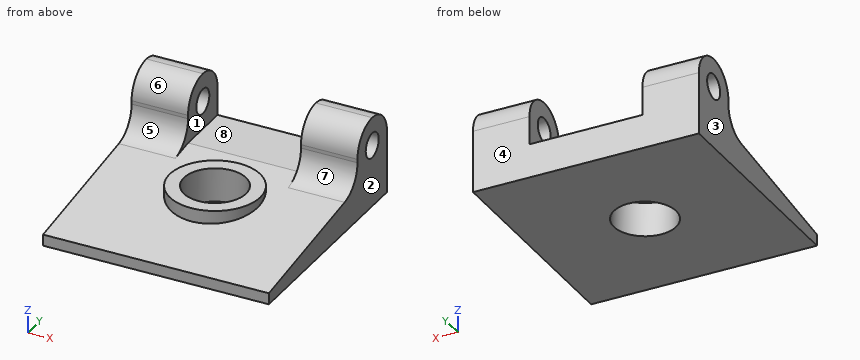
from build123d import *

# Parameters (mm, degrees)
F0_W        = 20
F0_H        = 20
F0_R        = 4
F1_DEPTH    = 4
F1_FACE_W   = 20
F1_FACE_H   = 20
F1_FACE_R   = 4
F0_R_2      = 2.75
F2_DEPTH    = 1
F3_W        = 5
F3_H        = 5
F4_DEPTH    = 5
F5_T1_DEPTH = 97.9746917615
F6_R        = 2.49999
F7_R        = 1.1
F8_DEPTH    = 25
F9_DEPTH    = 5
F10_DEPTH   = 2
F11_DEPTH   = 2


# Not quite as in the source:
# - a fillet or chamfer that OpenCascade refuses, or shapes differently, is made with other operations: its cross-section is extruded or revolved along the edge and cut away or added
# - a fillet or chamfer is up to 0.001 mm smaller than in the source, because OpenCascade refuses the exact size


with BuildPart() as f1:
    # F0 (on Top) → F1 (new body)
    with BuildSketch(Plane.XY):
        with Locations((10, 10)):
            Rectangle(F0_W, F0_H)
        with Locations((10, 10)):
            Circle(F0_R, mode=Mode.SUBTRACT)
    extrude(amount=F1_DEPTH)

    # F1_face (on face) + F0 (on Top) → F2 (join)
    with BuildSketch(Plane(origin=(10, 10, 4), x_dir=(1, 0, 0), z_dir=(0, 0, 1))):
        Rectangle(F1_FACE_W, F1_FACE_H)
        Circle(F1_FACE_R, mode=Mode.SUBTRACT)
    with BuildSketch(Plane.XY):
        with Locations((10, 10)):
            Circle(F0_R)
        with Locations((10, 10)):
            Circle(F0_R_2, mode=Mode.SUBTRACT)
    extrude(amount=F2_DEPTH)

    # F3 (on face) → F4 (join)
    with BuildSketch(Plane.XY.offset(5)):
        with Locations((2.5, 17.5)):
            Rectangle(F3_W, F3_H)
        with Locations((17.5, 17.5)):
            Rectangle(F3_W, F3_H)
    extrude(amount=F4_DEPTH)

    # F5: chamfer of 15 x 2 on 1 edges, made by hand

    # F5_s2 → F5_t1 (cut)
    with BuildSketch(Plane.YZ.offset(-38.9873458808)):
        Polygon((0, 3), (15, 5), (0, 5), align=None)
    extrude(amount=F5_T1_DEPTH, mode=Mode.SUBTRACT)

    # F6 (radius 2.5 in the source; OpenCascade refuses exactly that, so slightly less here)
    f6_edges = [f1.edges().sort_by_distance(p)[0] for p in [
        (2.5, 15, 5),
        (2.5, 15, 10),
        (17.5, 15, 5),
        (17.5, 15, 10),
        (2.5, 20, 10),
        (17.5, 20, 10),
    ]]
    fillet(f6_edges, radius=F6_R)

    # F7 (on face) → F8 (cut)
    with BuildSketch(Plane(origin=(0, 0, 0), x_dir=(0, -1, 0), z_dir=(-1, 0, 0))):
        with Locations((-17.5, 7.5)):
            Circle(F7_R)
    extrude(amount=-F8_DEPTH, mode=Mode.SUBTRACT)

    # F0 (on Top) → F9 (join)
    with BuildSketch(Plane.XY):
        with Locations((10, 10)):
            Circle(F0_R)
        with Locations((10, 10)):
            Circle(F0_R_2, mode=Mode.SUBTRACT)
    extrude(amount=F9_DEPTH)

    # F0 (on Top) → F10 (join)
    with BuildSketch(Plane.XY):
        with Locations((10, 10)):
            Circle(F0_R_2)
    extrude(amount=F10_DEPTH)

    # F0 (on Top) → F11 (cut)
    with BuildSketch(Plane.XY):
        with Locations((10, 10)):
            Rectangle(F0_W, F0_H)
        with Locations((10, 10)):
            Circle(F0_R, mode=Mode.SUBTRACT)
        with Locations((10, 10)):
            Circle(F0_R)
        with Locations((10, 10)):
            Circle(F0_R_2, mode=Mode.SUBTRACT)
        with Locations((10, 10)):
            Circle(F0_R_2)
    extrude(amount=F11_DEPTH, mode=Mode.SUBTRACT)


solid = f1.part
CAD build for the part. Positions are in the model's coordinates, mm. Face numbers are marked on the shaded views. A direction names the side the tool comes from. Give positions to 0.01 mm unless a question says otherwise; leave off trailing zeros. Order: outer loops, then holes, each group sorted by start corner. A loop starts at its lowest first (then second) coordinate and runs counter-clockwise, first axis right, second up. Notation, with made-up numbers: (71.5, 64) - (129.5, 64) arc R20 cw to (129.5, 90) - close; hole circle Ø3 at (41.25, 86.25). An arc over 180 degrees is marked (long way). Answer in a Markdown table with one row per item.
1. Flat gauge pin, fed straight in: pin 1 (4 mm diameter, centred on x = 8, y = 18.5, fed in from +Z). Where does the tip first touch, or does it go through?
Data:
| item | result |
|---|---|
| pin 1 | stops at z = 5 |
2. Pull direction X, two halves, no side cores. Call the marked faces 1, 2, 3 and 4: pulls with the +X half, pulls with the -X half, needs draft (parallel to the pull), parting line crosses it, or undercut.
Data:
| item | result |
|---|---|
| face 1 | undercut |
| face 2 | pulls with the +X half |
| face 3 | pulls with the -X half |
| face 4 | needs draft |
3. Saw through at A-A, the plane z = 5.5. Give the cut face in (x, y).
Data:
| item | result |
|---|---|
| outline | (0, 14.34) - (5, 14.34) - (5, 20) - (0, 20) - close; (15, 14.34) - (20, 14.34) - (20, 20) - (15, 20) - close |
4. Saw through at B-B, the plane x = 10. Give the cut face in (y, z), plus the area to 3 significant figures.
Data:
| item | result |
|---|---|
| outline | (0, 2) - (7.25, 2) - (7.25, 5) - (6, 5) - (6, 3.8) - (0, 3) - close; (12.75, 2) - (20, 2) - (20, 5) - (15, 5) - (14, 4.87) - (14, 5) - (12.75, 5) - close |
| area | 33.8 mm² |
5. Tool access for the marked faces 5, 6, 7 and 8: list every direction of +Z, -Z, +X, -X, +Y, -Y with a clear straight run to the whole face (end or side of a thin tool).
Data:
| item | result |
|---|---|
| face 5 | +Z, -X, -Y |
| face 6 | +Z, +X, -X, -Y |
| face 7 | +Z, +X, -Y |
| face 8 | +Z, +Y, -Y |
6. Probe probe 1 along Z at (x, y) = (18.85, 17.5); probe 2 along Y at (x, z) = (10, 4.3); probe 3 along Z at (x, y) = (11.75, 13.5). List the from-to ranges inside material, lowest first. Write a range as [from, to].
Data:
| item | result |
|---|---|
| probe 1 | z = [2, 6.4], [8.6, 10] |
| probe 2 | y = [6, 7.25], [12.75, 20] |
| probe 3 | z = [2, 5] |
7. Saw through at C-C, the plane z = 6.75. Give the cut face in (x, y), plus the area to 3 significant figures.
Data:
| item | result |
|---|---|
| outline | (0, 14.96) - (5, 14.96) - (5, 16.7) - (0, 16.7) - close; (0, 18.3) - (5, 18.3) - (5, 20) - (0, 20) - close; (15, 14.96) - (20, 14.96) - (20, 16.7) - (15, 16.7) - close; (15, 18.3) - (20, 18.3) - (20, 20) - (15, 20) - close |
| area | 34.3 mm² |
